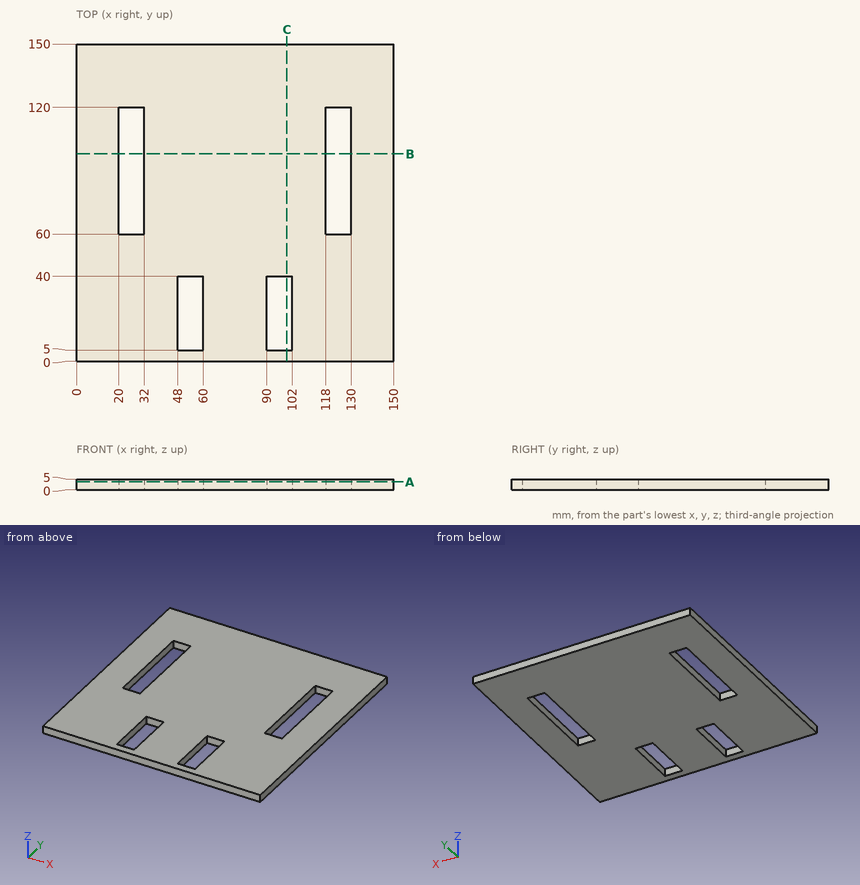
Part print with two shaded views. Sizes in mm from the minimum x, y, z corner. Round coordinates to 2 decimals unless told otherwise and drop trailing zeros. Order: outer loops, then holes, each group sorted by start corner. A loop starts at its lowest first (then second) coordinate and runs counter-clockwise, first axis right, second up. Notation, with made-up numbers: (11, 43.25) - (27, 43.25) arc R12 cw to (27, 47.25) - close; hole circle Ø6 at (3.25, -5.75). An arc over 180 degrees is marked (long way). Answer in a Markdown table with one row per item. Add a question column.
(1) Band-saw the part on A-A on z = 3.65. List the corners of the cut face in (x, y), and give its area (3 significant figures).
(2) Band-saw the part on B-B on y = 98. List the corners of the cut face in (x, z), and give its area (3 significant figures).
(3) Drop a flat-ended pin along its axis: pin 1 Ø2.5 at (y, z) = (24, 2) entering from -X. Give the stop position or say it passes through.
(4) Band-saw the part on C-C on x = 99.5. List the corners of the cut face in (y, z).
(5) Probe L1, parallel to X at y = 71, z = 4.3; L2, parallel to X at y = 17, z = 0.65; L3, parallel to Y at x = 21, z = 0.5. List the from-to ranges inside material, lowest first. Write a range as [from, to].
Data:
| question | item | result |
|---|---|---|
| 1 | outline | (0, 0) - (150, 0) - (150, 150) - (0, 150) - close; hole (20, 60) - (32, 60) - (32, 120) - (20, 120) - close; hole (48, 5) - (60, 5) - (60, 40) - (48, 40) - close; hole (90, 5) - (102, 5) - (102, 40) - (90, 40) - close; hole (118, 60) - (130, 60) - (130, 120) - (118, 120) - close |
| 1 | area | 20,200 mm^2 |
| 2 | outline | (0, 0) - (20, 0) - (20, 5) - (0, 5) - close; (32, 0) - (118, 0) - (118, 5) - (32, 5) - close; (130, 0) - (150, 0) - (150, 5) - (130, 5) - close |
| 2 | area | 630 mm^2 |
| 3 | pin 1 | stops at x = 0 |
| 4 | outline | (0, 0) - (5, 0) - (5, 5) - (0, 5) - close; (40, 0) - (150, 0) - (150, 5) - (40, 5) - close |
| 5 | L1 | x = [0, 20], [32, 118], [130, 150] |
| 5 | L2 | x = [0, 48], [60, 90], [102, 150] |
| 5 | L3 | y = [0, 60], [120, 150] |
